Geometry check sheet. Reference: the model listing, model coordinates, mm. Round coordinates to 2 decimals unless told otherwise and drop trailing zeros. Order: outer loops, then holes, each group sorted by start corner. A loop starts at its lowest first (then second) coordinate and runs counter-clockwise, first axis right, second up.
(1) Go/stop test with a flat-tipped pin: pin 1 (5 mm diameter, centred on x = -37.338, z = 18.542, fed in from +Y). Record where the tip stops, or that it passes through.
(2) Material ranges on line 1 along X through (y, z) = (3.4, 38.1); line 2 along X through (y, z) = (1.7, 17.5); line 3 along Z through (x, y) = (36.5, 1.9), recorded low to high.
(3) Sectioned sample at A-A (z = 38.1). Record the boundary of the cut face in (x, y), plus the area to 3 significant figures.
Autodesk Inventor part; units mm, degrees
ref_plane "YZ Plane" through (0, 0, 0) normal (1, 0, 0) x (0, 1, 0)
ref_plane "XZ Plane" through (0, 0, 0) normal (0, 1, 0) x (-1, 0, 0)
ref_plane "XY Plane" through (0, 0, 0) normal (0, 0, 1) x (1, 0, 0)
sketch "Sketch1" plane through (0, 0, 0) normal (0, 1, 0) x (-1, 0, 0)
  line L0 (-50.8, 63.5) -> (50.8, 63.5)
  line L1 (50.8, 63.5) -> (50.8, -63.5)
  line L2 (50.8, -63.5) -> (-50.8, -63.5)
  line L3 (-50.8, -63.5) -> (-50.8, 63.5)
  line L4 (-50.8, 63.5) -> (50.8, -63.5) construction
  line L5 (50.8, 63.5) -> (-50.8, -63.5) construction
  point P0 (0, 0)
  point P1 (0, 0)
  dimension "d0" = 101.6
  dimension "d1" = 127
extrude "Plate1" add sketch "Sketch1" along normal blind 5.08
sketch "Sketch2" plane through (0, 5.08, 0) normal (0, 1, 0) x (1, 0, 0)
  line L0 (-50.8, 63.5) -> (50.8, 63.5) construction
  line L1 (0, 63.5) -> (0, -63.5) construction
  line L2 (50.8, -63.5) -> (-50.8, -63.5) construction
  line L3 (-50.8, -63.5) -> (-50.8, 63.5) construction
  point P0 (0, 0)
  point P1 (-37.338, -38.1)
  point P2 (-37.338, -18.542)
  point P3 (37.338, -38.1)
  point P4 (37.338, -18.542)
  dimension "d5" = 19.558
  dimension "d6" = 13.462
  dimension "d14" = 25.4
hole "Hole1" at (-37.338, 5.08, 38.1) at (-37.338, 5.08, 18.542) at (37.338, 5.08, 38.1) at (37.338, 5.08, 18.542) direction (0, -1, 0) diameter 3.2766 end through all
sketch "Sketch3" plane through (0, 5.08, 0) normal (0, 1, 0) x (1, 0, 0)
  line L0 (0, 0) -> (0, 25.4) construction
  point P0 (-6.604, 56.8607)
  point P1 (6.604, 56.8607)
  dimension "d15" = 25.4
  dimension "d16" = 13.208
hole "Hole2" at (-6.604, 5.08, -56.8607) at (6.604, 5.08, -56.8607) direction (0, -1, 0) diameter 2.286 end through all
equation "\"d12\" = Thickness"
equation "\"d22\" = Thickness"
equation "\"d4\" = Thickness"
equation "\"BendRadius\" = Thickness"
equation "\"BendReliefWidth\" = Thickness"
equation "\"BendReliefDepth\" = 0.5 * Thickness"
equation "\"CornerReliefSize\" = 4 * Thickness"
equation "\"MinimumRemnant\" = 2 * Thickness"
equation "\"TransitionRadius\" = BendRadius"
equation "\"JacobiRadiusSize\" = BendRadius"
equation "\"GapSize\" = Thickness"
equation "\"motor_placement\" = 25.4"
properties part number "pibot_baseplate" material "Polycarbonate, Clear"
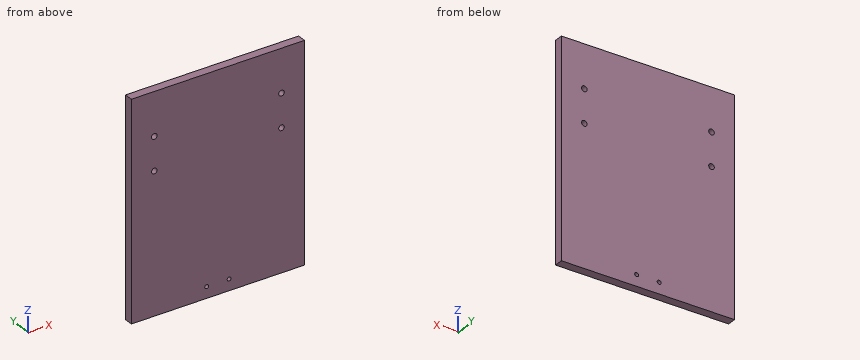
Answer below:
1. pin 1: stops at y = 5.08
2. line 1: x = -50.8 to -38.98, -35.7 to 35.7, 38.98 to 50.8
2. line 2: x = -50.8 to -38.6, -36.07 to 36.07, 38.6 to 50.8
2. line 3: z = -63.5 to 17.13, 19.95 to 36.69, 39.51 to 63.5
3. outline: (-50.8, 0) - (-38.98, 0) - (-38.98, 5.08) - (-50.8, 5.08) - close; (-35.7, 0) - (35.7, 0) - (35.7, 5.08) - (-35.7, 5.08) - close; (38.98, 0) - (50.8, 0) - (50.8, 5.08) - (38.98, 5.08) - close
3. area: 483 mm2
